Work out the finished part from the listing and answer in its coordinate system (mm). Face numbers are marked on the shaded views. A direction names the side the tool comes from. Round coordinates to 2 decimals unless told otherwise and drop trailing zeros. Order: outer loops, then holes, each group sorted by start corner. A loop starts at its lowest first (then second) coordinate and runs counter-clockwise, first axis right, second up. Notation, with made-up numbers: (-23, 8.25) - (10, 8.25) arc R18 ccw to (10, 30.25) - close; hole circle Ø6 at (67.25, 4.25). An arc over 180 degrees is marked (long way). Use CSV: the item, a comma, the result in double quotes.
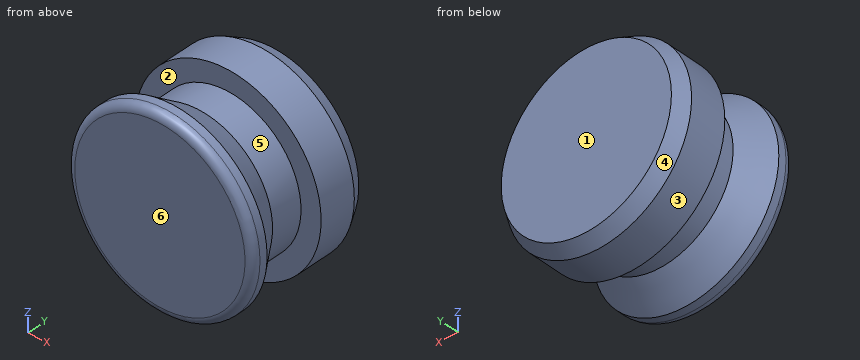
from build123d import *

# Parameters (mm, degrees)
FILLET1_R      = 0.79375
CHAMFER1_SIZE  = 0.79375
CHAMFER1_SIZE2 = 1.374815329


with BuildPart() as part:
    # Sketch1 → Revolve1 (revolve)
    with BuildSketch(Plane.XY):
        Polygon((0, 0), (-9.398, 0), (-9.398, 1.5875), (-7.366, 4.445), (-7.366, 7.62), (-9.398, 7.62), (-9.398, 12.7), (0, 12.7), align=None)
    revolve(axis=Axis((0, 0, 0), (0, 1, 0)))

    # Fillet1
    fillet1_edges = [part.edges().sort_by_distance(p)[0] for p in [
        (9.398, 0, 0),
    ]]
    fillet(fillet1_edges, radius=FILLET1_R)

    # Chamfer1
    chamfer1_edges = [part.edges().sort_by_distance(p)[0] for p in [
        (9.398, 12.7, 0),
    ]]
    chamfer1_side = [part.faces().sort_by_distance(p)[0] for p in [
        (0, 12.7, 0),
    ]]
    chamfer(chamfer1_edges, length=CHAMFER1_SIZE, length2=CHAMFER1_SIZE2, reference=chamfer1_side[0])


solid = part.part
(1) Find section C-C (y = 7.25). Determine the outline of the cut face in (x, z).
Findings below:
outline,"circle Ø14.73 at (0, 0)"
(2) Each of these flat-tipped pins is pushed along its axis until it touches: pin 1 (10 mm diameter, centred on x = 0, z = -7, fed in from -Y); pin 2 (1.5 mm diameter, centred on y = 7.5, z = 4, fed in from +X). Where does it stop, or does it pass through?
Findings below:
pin 1,"stops at y = 0"
pin 2,"stops at x = 8.81"
(3) Find the intervals of material crossed by L1, parallel to Y at x = 4.75, z = -6.75; L2, parallel to Y at x = 8.5, z = -0.25; L3, parallel to Z at x = 0, y = 9, in increasing order. Write a range as from..to.
Findings below:
L1,"y = 0..3.2, 7.62..12.7"
L2,"y = 0..2.85, 7.62..12.7"
L3,"z = -9.4..9.4"
(4) The mould has two halves that part along Y. Classify the marked faces 3, 4, 5 and 6: released by +Y, released by -Y, zero draft, split by the parting line, or undercut.
Findings below:
face 3,"zero draft"
face 4,"released by +Y"
face 5,"undercut"
face 6,"released by -Y"
(5) Find section B-B (x = 0). Determine the outline of the cut face in (y, z) (1 decimal), and give its area (3 significant figures).
Findings below:
outline,"(0, -8.6) arc R0.8 ccw to (0.8, -9.4) - (1.6, -9.4) - (4.4, -7.4) - (7.6, -7.4) - (7.6, -9.4) - (11.3, -9.4) - (12.7, -8.6) - (12.7, 8.6) - (11.3, 9.4) - (7.6, 9.4) - (7.6, 7.4) - (4.4, 7.4) - (1.6, 9.4) - (0.8, 9.4) arc R0.8 ccw to (0, 8.6) - close"
area,"219 mm²"
(6) For the marked faces 1 and 2, determine the directions among +Z, -Z, +X, -X, +Y, -Y from which every point of the face is accessible in a straight line to the end or side of a thin tool.
Findings below:
face 1,"+Z, -Z, +X, -X, +Y"
face 2,"none"
(7) Find section A-A (z = 0). Determine the outline of the cut face in (x, y) (1 decimal).
Findings below:
outline,"(-9.4, 0.8) arc R0.8 ccw to (-8.6, 0) - (8.6, 0) arc R0.8 ccw to (9.4, 0.8) - (9.4, 1.6) - (7.4, 4.4) - (7.4, 7.6) - (9.4, 7.6) - (9.4, 11.3) - (8.6, 12.7) - (-8.6, 12.7) - (-9.4, 11.3) - (-9.4, 7.6) - (-7.4, 7.6) - (-7.4, 4.4) - (-9.4, 1.6) - close"
